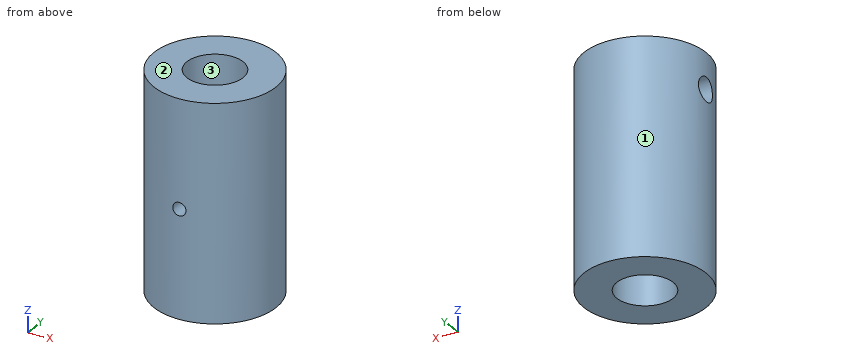
```python
from build123d import *

# Parameters (mm, degrees)
SKETCH2_R               = 32.512
SKETCH2_R_2             = 15
BOSS_EXTRUDE1_DEPTH     = 57.15
CUT_EXTRUDE1_REACH      = 75.35
CUT_EXTRUDE1_END_RADIUS = 32.512
SKETCH3_R               = 6.35
CUT_EXTRUDE2_REACH      = 75.35
CUT_EXTRUDE2_END_RADIUS = 32.512
SKETCH5_R               = 3.5


with BuildPart() as part:
    # Sketch2 → Boss-Extrude1 (new, symmetric)
    with BuildSketch(Plane.XY):
        Circle(SKETCH2_R)
        Circle(SKETCH2_R_2, mode=Mode.SUBTRACT)
    extrude(amount=BOSS_EXTRUDE1_DEPTH, both=True)

    # Cut-Extrude1: up to this cylinder (the profile starts inside it)
    cut_extrude1_end = Plane(origin=(0, 0, 38.1), z_dir=(0, 0, -1)) * Cylinder(CUT_EXTRUDE1_END_RADIUS, 216.724, mode=Mode.PRIVATE)
    # Sketch3 → Cut-Extrude1 (cut, up to the surface)
    with BuildSketch(Plane(origin=(0, 0, 0), x_dir=(0, 0, -1), z_dir=(1, 0, 0)), mode=Mode.PRIVATE) as cut_extrude1_sk1:
        with Locations((-38.1, 0)):
            Circle(SKETCH3_R)
    cut_extrude1_tool1 = extrude(cut_extrude1_sk1.sketch, amount=-CUT_EXTRUDE1_REACH, mode=Mode.PRIVATE) & cut_extrude1_end
    add(cut_extrude1_tool1.solids().sort_by_distance((0, 0, 38.1))[0], mode=Mode.SUBTRACT)

    # Cut-Extrude2: up to this cylinder (the profile starts inside it)
    cut_extrude2_end = Plane(origin=(0, 0, 0), z_dir=(0, 0, -1)) * Cylinder(CUT_EXTRUDE2_END_RADIUS, 216.724, mode=Mode.PRIVATE)
    # Sketch5 → Cut-Extrude2 (cut, up to the surface)
    with BuildSketch(Plane(origin=(0, 0, 0), x_dir=(1, 0, 0), z_dir=(0, 1, 0)), mode=Mode.PRIVATE) as cut_extrude2_sk1:
        with Locations(Location((0, 0, 0), (0, 0, 270))):
            Circle(SKETCH5_R)
    cut_extrude2_tool1 = extrude(cut_extrude2_sk1.sketch, amount=-CUT_EXTRUDE2_REACH, mode=Mode.PRIVATE) & cut_extrude2_end
    add(cut_extrude2_tool1.solids().sort_by_distance((0, 0, 0))[0], mode=Mode.SUBTRACT)


solid = part.part
```
Source: CAD feature listing. Evaluate the final solid. Frame: model axes, mm. Face numbers are marked on the shaded views. Round coordinates to 2 decimals unless told otherwise and drop trailing zeros. Loops run counter-clockwise (first coordinate to the right, second up) from the corner with the lowest first, then second, coordinate; pieces in that order, holes last.
(1) Section query A-A (x = 0). Output: boundary loops of the cut face in (y, z), and give its area (3 significant figures).
From the geometry:
outline: (-32.51, -57.15) - (-15, -57.15) - (-15, -3.5) - (-32.51, -3.5) - close; (-32.51, 3.5) - (-15, 3.5) - (-15, 57.15) - (-32.51, 57.15) - close; (15, -57.15) - (32.51, -57.15) - (32.51, 57.15) - (15, 57.15) - close
area: 3,880 mm2
(2) Section query D-D (y = -17.5). Output: boundary loops of the cut face in (x, z), and give its area (3 significant figures).
From the geometry:
outline: (-27.4, -57.15) - (27.4, -57.15) - (27.4, 57.15) - (-27.4, 57.15) - close; hole circle Ø7 at (0, 0)
area: 6,230 mm2
(3) Pull-direction query (Y, two-part tool) for the marked faces 1, 2 and 3; classes: +Y half, -Y half, draft (parallel to the pull), parting line (faces both ways), or undercut.
From the geometry:
face 1: parting line
face 2: draft
face 3: undercut
(4) Section query C-C (y = -9). Output: boundary loops of the cut face in (x, z).
From the geometry:
outline: (-31.24, -57.15) - (-12, -57.15) - (-12, 57.15) - (-31.24, 57.15) - close; (12, -57.15) - (31.24, -57.15) - (31.24, 57.15) - (12, 57.15) - close
(5) Section query B-B (y = 0). Output: boundary loops of the cut face in (x, z).
From the geometry:
outline: (-32.51, -57.15) - (-15, -57.15) - (-15, 31.75) - (-32.51, 31.75) - close; (-32.51, 44.45) - (-15, 44.45) - (-15, 57.15) - (-32.51, 57.15) - close; (15, -57.15) - (32.51, -57.15) - (32.51, 57.15) - (15, 57.15) - close
(6) Material intervals for probe 1 along Z at (x, y) = (0, -19.75); probe 2 along Y at (x, z) = (0, 5); probe 3 along X at (y, z) = (-5, -12.5), sorted ascending.
From the geometry:
probe 1: z = -57.15 to -3.5, 3.5 to 57.15
probe 2: y = -32.51 to -15, 15 to 32.51
probe 3: x = -32.13 to -14.14, 14.14 to 32.13
(7) Contact query for flat-ended pins moving along their axis: pin 1 Ø6.5 at (x, z) = (0, 0) entering from -Y; pin 2 Ø12 at (x, z) = (-3.5, 40.5) entering from -Y; pin 3 Ø1.5 at (y, z) = (10.5, 27.5) entering from +X. Output: stop coordinate, or through.
From the geometry:
pin 1: stops at y = 14.64
pin 2: stops at y = -32.51
pin 3: stops at x = 31.02
